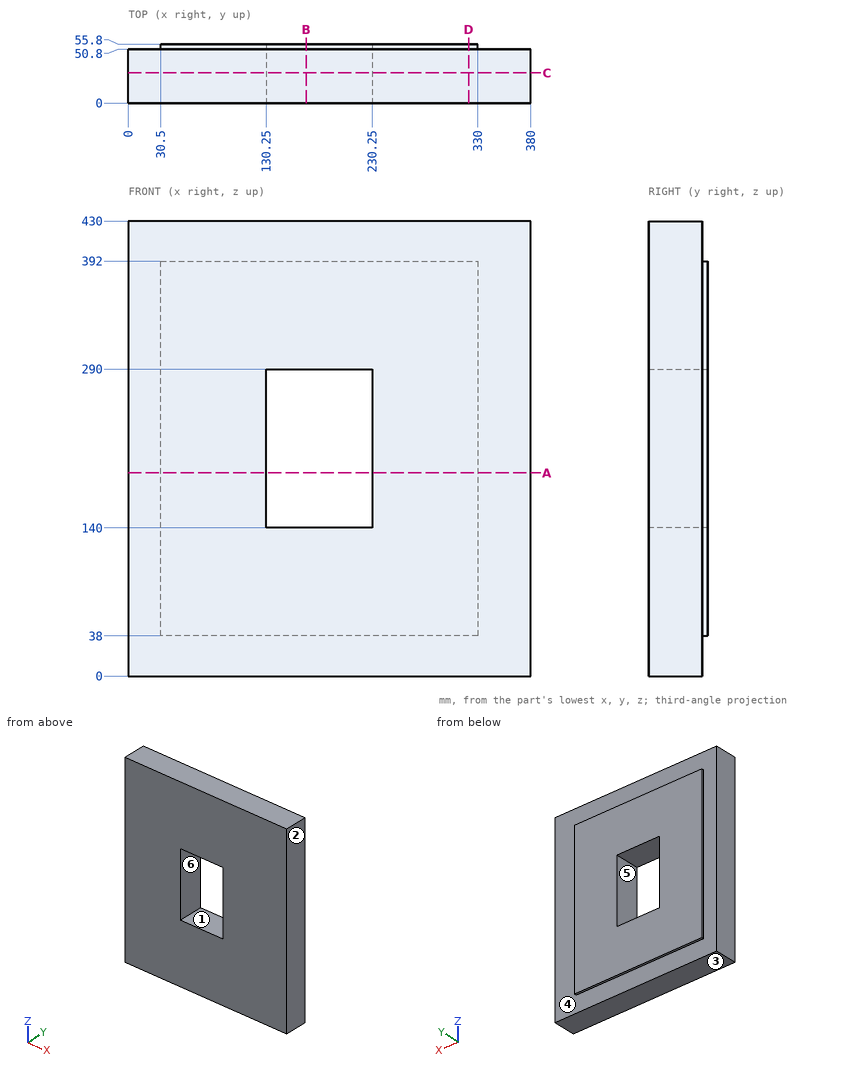
Drawing for the job (mm, zero at the part's lowest x, y, z). A direction names the side the tool comes from. Coordinates: 2 decimals unless noted, no trailing zeros. Order: outer loops, then holes, each group sorted by start corner. A loop starts at its lowest first (then second) coordinate and runs counter-clockwise, first axis right, second up. Notation, with made-up numbers: (-24.5, 9) - (-0.5, 9) arc R33 ccw to (-0.5, 43) - close; hole circle Ø2 at (31, 56.5). An arc over 180 degrees is marked (long way). Use a Markdown table: item, result. Add a question column.
(1) Flat gauge pins, fed straight in: pin 1 (4 mm diameter, centred on x = 243, y = 53.5, fed in from -Z); pin 2 (1.5 mm diameter, centred on x = 110, y = 52, fed in from +Z); pin 3 (4 mm diameter, centred on y = 53.5, z = 154, fed in from +X). Where does each tip first touch, or does it go through?
(2) Saw through at A-A (z = 192). Give the cut face in (x, y), then the cut area to 3 significant figures.
(3) Drill centre lines: line 1 along X through (y, z) = (40, 163.5); line 2 along X through (y, z) = (51, 206.5); line 3 along Z through (x, y) = (170, 22.5). Where is each one in solid material? Low to high. Write a range as [from, to].
(4) Which spindle directions (+Z, -Z, +X, -X, +Y, -Y) get a long thin tool onto all of the face, cutting with end or side? Do the marked faces 1 and 2. Say none if no direction does.
(5) Saw through at B-B (x = 168). Give the cut face in (y, z).
(6) Saw through at C-C (y = 28.5). Give the cut face in (x, z).
(7) Pull direction Z, two halves, no side cores. Call the marked faces 3, 4, 5 and 6: +Z half, -Z half, draft (parallel to the pull), parting line (faces both ways), or undercut.
(8) Saw through at D-D (x = 321.5). Give the cut face in (y, z).
Solved:
| question | item | result |
|---|---|---|
| 1 | pin 1 | stops at z = 38 |
| 1 | pin 2 | stops at z = 392 |
| 1 | pin 3 | stops at x = 330 |
| 2 | outline | (0, 0) - (130.25, 0) - (130.25, 55.8) - (30.5, 55.8) - (30.5, 50.8) - (0, 50.8) - close; (230.25, 0) - (380, 0) - (380, 50.8) - (330, 50.8) - (330, 55.8) - (230.25, 55.8) - close |
| 2 | area | 15,200 mm² |
| 3 | line 1 | x = [0, 130.25], [230.25, 380] |
| 3 | line 2 | x = [30.5, 130.25], [230.25, 330] |
| 3 | line 3 | z = [0, 140], [290, 430] |
| 4 | face 1 | +Y, -Y |
| 4 | face 2 | +Z, -Z, +X, +Y, -Y |
| 5 | outline | (0, 0) - (50.8, 0) - (50.8, 38) - (55.8, 38) - (55.8, 140) - (0, 140) - close; (0, 290) - (55.8, 290) - (55.8, 392) - (50.8, 392) - (50.8, 430) - (0, 430) - close |
| 6 | outline | (0, 0) - (380, 0) - (380, 430) - (0, 430) - close; hole (130.25, 140) - (230.25, 140) - (230.25, 290) - (130.25, 290) - close |
| 7 | face 3 | -Z half |
| 7 | face 4 | draft |
| 7 | face 5 | undercut |
| 7 | face 6 | undercut |
| 8 | outline | (0, 0) - (50.8, 0) - (50.8, 38) - (55.8, 38) - (55.8, 392) - (50.8, 392) - (50.8, 430) - (0, 430) - close |
